Verification items for the finished model (mm, model axes). A direction names the side the tool comes from. Coordinates: 2 decimals unless noted, no trailing zeros. Loops run counter-clockwise (first coordinate to the right, second up) from the corner with the lowest first, then second, coordinate; pieces in that order, holes last. Notation, with made-up numbers: M 22,23.25 L 80,23.25 A13 cw 80,40.25 Z; hole C 42.25,14.5 d1. An arc over 180 degrees is marked long. Write item = value, one per line. Start each with the question number.
```python
from build123d import *

# Parameters (mm, degrees)
CROQUIS1_W                 = 70
CROQUIS1_H                 = 15.6
SALIENTE_EXTRUIR1_DEPTH    = 4
CORTAR_EXTRUIR2_DEPTH      = 37.081019941
CORTAR_EXTRUIR2_DEPTH_BACK = 37.081019941
CROQUIS3_R                 = 3.2
CROQUIS3_R_2               = 2.2
REDONDEO1_R                = 4
CORTAR_EXTRUIR4_DEPTH      = 3.2


with BuildPart() as part:
    # Croquis1 → Saliente-Extruir1 (new body)
    with BuildSketch(Plane(origin=(0, 0, 0), x_dir=(1, 0, 0), z_dir=(0, 1, 0))):
        Rectangle(CROQUIS1_W, CROQUIS1_H)
    extrude(amount=SALIENTE_EXTRUIR1_DEPTH)

    # Croquis3 → Cortar-Extruir2 (cut, two sides: drawn at the far end of the back side and taken through both)
    with BuildSketch(Plane(origin=(0, 0, 0), x_dir=(1, 0, 0), z_dir=(0, 1, 0)).offset(-CORTAR_EXTRUIR2_DEPTH_BACK)):
        with Locations(Location((0, 0, 0), (0, 0, 90))):
            Circle(CROQUIS3_R)
        with Locations(Location((20, 0, 0), (0, 0, 90))):
            Circle(CROQUIS3_R_2)
        with Locations(Location((-20, 0, 0), (0, 0, 90))):
            Circle(CROQUIS3_R_2)
    extrude(amount=CORTAR_EXTRUIR2_DEPTH + CORTAR_EXTRUIR2_DEPTH_BACK, mode=Mode.SUBTRACT)

    # Redondeo1
    redondeo1_edges = [part.edges().sort_by_distance(p)[0] for p in [
        (35, 2, 7.8),
        (-35, 2, 7.8),
        (-35, 2, -7.8),
        (35, 2, -7.8),
    ]]
    fillet(redondeo1_edges, radius=REDONDEO1_R)

    # Croquis5 → Cortar-Extruir4 (cut)
    with BuildSketch(Plane(origin=(0, 0, 0), x_dir=(1, 0, 0), z_dir=(0, 1, 0))):
        Polygon((-15.727608008, 0), (-17.863804004, 3.7), (-22.136195996, 3.7), (-24.272391992, 0), (-22.136195996, -3.7), (-17.863804004, -3.7), align=None)
        Polygon((17.863804004, -3.7), (15.727608008, 0), (17.863804004, 3.7), (22.136195996, 3.7), (24.272391992, 0), (22.136195996, -3.7), align=None)
    extrude(amount=CORTAR_EXTRUIR4_DEPTH, mode=Mode.SUBTRACT)


solid = part.part
```
Q1. Gauge pin test, flat end, axial feed: pin 1 (3.5 mm diameter, centred on x = 19, z = 0, fed in from -Y). Record the tip position at first contact, or that the pin passes through.
Q2. Mould release check, pull along Z, two halves, no side actions. Record for faces 3 (the face through (16.811, 1.578, 1.876)), 4 (the face through (-35, 2, 0)), 5 (the face through (33.797, 2.028, 6.659)): +Z half, -Z half, draft (parallel to the pull), parting line (faces both ways), or undercut.
Q3. Set-up check for faces 1 (the face through (-33.859, 2.028, -6.597)), 2 (the face through (20, 2, -3.7)): record each of +Z, -Z, +X, -X, +Y, -Y from which the full face is reachable in a straight line by a thin tool's end or side.
Q4. Sectioned sample at B-B on y = 2.35. Record the cut outline in (x, z).
Q5. Sectioned sample at C-C on z = 1.5. Record the cut outline in (x, y), plus the area to 3 significant figures.
Q6. Sectioned sample at A-A on x = 20. Record the cut outline in (y, z), plus the area to 3 significant figures.
Q7. Scan lines: L1, parallel to X at y = 1.2, z = 0; L2, parallel to X at y = 3.8, z = 0; L3, parallel to Z at x = -18, y = 2.4. Record each from-to range of solid material in increasing order. Write a range as [from, to].
Q8. Sectioned sample at D-D on x = 0. Record the cut outline in (y, z), plus the area to 3 significant figures.
Solutions:
q1.pin_1 = 3.2
q2.face_3 = undercut
q2.face_4 = draft
q2.face_5 = +Z half
q3.face_1 = -Z, -X, +Y, -Y
q3.face_2 = -Y
q4.outline = M -35,-3.8 A4 ccw -31,-7.8 L 31,-7.8 A4 ccw 35,-3.8 L 35,3.8 A4 ccw 31,7.8 L -31,7.8 A4 ccw -35,3.8 Z; hole M -24.27,0 L -22.14,-3.7 L -17.86,-3.7 L -15.73,0 L -17.86,3.7 L -22.14,3.7 Z; hole C 0,0 d6.4; hole M 15.73,0 L 17.86,-3.7 L 22.14,-3.7 L 24.27,0 L 22.14,3.7 L 17.86,3.7 Z
q5.outline = M -35,0 L -23.41,0 L -23.41,3.2 L -21.61,3.2 L -21.61,4 L -35,4 Z; M -18.39,3.2 L -16.59,3.2 L -16.59,0 L -2.83,0 L -2.83,4 L -18.39,4 Z; M 2.83,0 L 16.59,0 L 16.59,3.2 L 18.39,3.2 L 18.39,4 L 2.83,4 Z; M 21.61,3.2 L 23.41,3.2 L 23.41,0 L 35,0 L 35,4 L 21.61,4 Z
q5.area = 209 mm²
q6.outline = M 0,-7.8 L 4,-7.8 L 4,-2.2 L 3.2,-2.2 L 3.2,-3.7 L 0,-3.7 Z; M 0,3.7 L 3.2,3.7 L 3.2,2.2 L 4,2.2 L 4,7.8 L 0,7.8 Z
q6.area = 35.2 mm²
q7.L1 = [-35, -24.27], [-15.73, -3.2], [3.2, 15.73], [24.27, 35]
q7.L2 = [-35, -22.2], [-17.8, -3.2], [3.2, 17.8], [22.2, 35]
q7.L3 = [-7.8, -3.7], [3.7, 7.8]
q8.outline = M 0,-7.8 L 4,-7.8 L 4,-3.2 L 0,-3.2 Z; M 0,3.2 L 4,3.2 L 4,7.8 L 0,7.8 Z
q8.area = 36.8 mm²
